Here's how the part is built. I have some questions about the finished solid (model axes, mm). Face numbers are marked on the shaded views. A direction names the side the tool comes from. Give positions to 0.01 mm unless a question says otherwise; leave off trailing zeros. Write each loop counter-clockwise with the first axis right and the second up, starting at its lowest first coordinate (ties: lowest second). Pieces come first, ordered by that corner, then holes. Notation, with made-up numbers: M -14.75,-16 L -5.75,-16 A24 ccw -5.75,-4 Z; hole C 25,-21 d10. An arc over 180 degrees is marked long. Use one line per item in the form item = value. Start each with the question number.
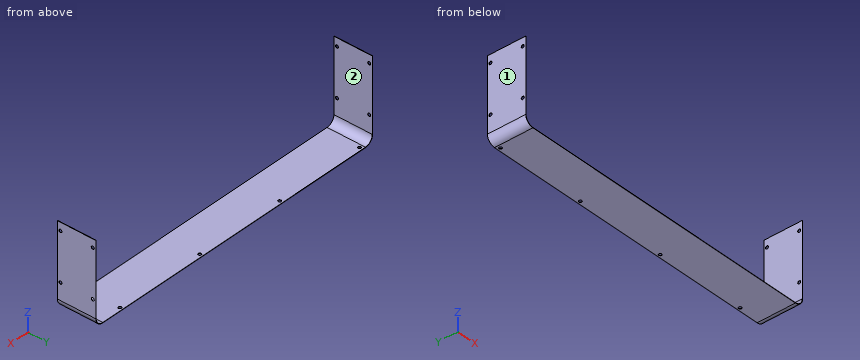
from build123d import *

# Parameters (mm, degrees)
BASE_FLANGE1_DEPTH = 76
SKETCH2_R          = 3
CUT_EXTRUDE1_DEPTH = 649.076816435
SKETCH3_R          = 3
CUT_EXTRUDE2_DEPTH = 10


# Read off the part's stored shape, not the designer's step: Base-Flange1
with BuildPart() as part:
    # Base-Flange1 outline → Base-Flange1 (new body)
    with BuildSketch(Plane(origin=(0, 0, 0), x_dir=(1, 0, 0), z_dir=(0, 1, 0))):
        with BuildLine():
            Line((622.7, 144), (622.7, 0))
            Line((622.7, 0), (623.4, 0))
            Line((623.4, 0), (623.4, 144))
            ThreePointArc((623.4, 144), (618.713708499, 155.313708499), (607.4, 160))
            Line((607.4, 160), (16, 160))
            ThreePointArc((16, 160), (4.686291501, 155.313708499), (0, 144))
            Line((0, 144), (0, 0))
            Line((0, 0), (0.7, 0))
            Line((0.7, 0), (0.7, 144))
            ThreePointArc((0.7, 144), (5.181266248, 154.818733752), (16, 159.3))
            Line((16, 159.3), (607.4, 159.3))
            ThreePointArc((607.4, 159.3), (618.218733752, 154.818733752), (622.7, 144))
        make_face()
    extrude(amount=BASE_FLANGE1_DEPTH)

    # Sketch2 → Cut-Extrude1 (cut, through all)
    with BuildSketch(Plane(origin=(623.4, 0, 0), x_dir=(0, 0, -1), z_dir=(1, 0, 0))):
        with Locations((16, 70)):
            Circle(SKETCH2_R)
        with Locations((111, 70)):
            Circle(SKETCH2_R)
        with Locations(Location((111, 6, 0), (0, 0, 180))):
            Circle(SKETCH2_R)
        with Locations(Location((16, 6, 0), (0, 0, 180))):
            Circle(SKETCH2_R)
    extrude(amount=-CUT_EXTRUDE1_DEPTH, mode=Mode.SUBTRACT)

    # Sketch3 → Cut-Extrude2 (cut)
    with BuildSketch(Plane(origin=(0, 0, -160), x_dir=(-1, 0, 0), z_dir=(0, 0, -1))):
        with Locations((-562.4, 70)):
            Circle(SKETCH3_R)
        with Locations((-382.4, 70)):
            Circle(SKETCH3_R)
        with Locations((-202.4, 70)):
            Circle(SKETCH3_R)
        with Locations((-22.4, 70)):
            Circle(SKETCH3_R)
        with Locations((157.6, 70)):
            Circle(SKETCH3_R)
        with Locations((337.6, 70)):
            Circle(SKETCH3_R)
        with Locations((517.6, 70)):
            Circle(SKETCH3_R)
        with Locations((-382.4, -22)):
            Circle(SKETCH3_R)
        with Locations((-202.4, -22)):
            Circle(SKETCH3_R)
        with Locations((-22.4, -22)):
            Circle(SKETCH3_R)
        with Locations((157.6, -22)):
            Circle(SKETCH3_R)
        with Locations((337.6, -22)):
            Circle(SKETCH3_R)
        with Locations((517.6, -22)):
            Circle(SKETCH3_R)
        with Locations((-562.4, -22)):
            Circle(SKETCH3_R)
    extrude(amount=-CUT_EXTRUDE2_DEPTH, mode=Mode.SUBTRACT)


solid = part.part
1) Suppose I cut it at C-C, the plane x = 397.5. List the corners of the cut face in (y, z) for me.
2) Please list where these lines run through material, in increasing order: line 1 (Y direction, x = 0.3, z = -111); line 2 (X direction, y = 62, z = -94); line 3 (Y direction, x = 22.4, z = -159.45).
3) Suppose I cut it at A-A, the plane z = -136. List the corners of the cut face in (x, y) for me.
4) Will these pins go through, and if not, where does the flat tip stop? P1, Ø3.5, axis at x = 202.4, y = 70, coming from the -Z side; P2, Ø10, axis at x = 123, y = 46, coming from the +Z side.
5) On a 3-axis mill with a long thin cutter (end or side, diameter ignored), from which of +Z, -Z, +X, -X, +Y, -Y can I reach the whole of each face in a straight line? I mean the marked faces 1 and 2. Say none if no direction works.
6) Suppose I cut it at B-B, the plane y = 19.5. List the corners of the cut face in (x, z) for me.
Checks:
q1.outline = M 0,-160 L 76,-160 L 76,-159.3 L 0,-159.3 Z
q2.line_1 = 0 to 3, 9 to 67, 73 to 76
q2.line_2 = 0 to 0.7, 622.7 to 623.4
q2.line_3 = 0 to 67, 73 to 76
q3.outline = M 0,0 L 0.7,0 L 0.7,76 L 0,76 Z; M 622.7,0 L 623.4,0 L 623.4,76 L 622.7,76 Z
q4.P1 = through
q4.P2 = -159.3
q5.face_1 = +Z, -Z, -X, +Y, -Y
q5.face_2 = +Z, +Y, -Y
q6.outline = M 0,-144 A16 ccw 16,-160 L 607.4,-160 A16 ccw 623.4,-144 L 623.4,0 L 622.7,0 L 622.7,-144 A15.3 cw 607.4,-159.3 L 16,-159.3 A15.3 cw 0.7,-144 L 0.7,0 L 0,0 Z
